Can you work these out from the model? Positions are in its coordinate system, mm. Give positions to 0.01 mm unless a question says otherwise; leave off trailing zeros. Order: outer loops, then holes, each group sorted by start corner. A loop starts at its lowest first (then second) coordinate and runs counter-clockwise, first axis right, second up. Notation, with made-up numbers: M -26.5,50.5 L -13.5,50.5 A21 cw -13.5,80.5 Z; hole C 20,-12.5 d9. An arc over 180 degrees is marked long. Write each question's results on one line, items separated by ' | '.
from build123d import *

# Parameters (mm, degrees)
SKETCH1_W           = 152.4
SKETCH1_H           = 63.5
BOSS_EXTRUDE1_DEPTH = 6.35
CUT_EXTRUDE1_REACH  = 14.7
SKETCH2_R           = 9.525


with BuildPart() as part:
    # Sketch1 → Boss-Extrude1 (new body, symmetric)
    with BuildSketch(Plane(origin=(0, 0, 0), x_dir=(0, 0, -1), z_dir=(1, 0, 0))):
        Rectangle(SKETCH1_W, SKETCH1_H)
    extrude(amount=BOSS_EXTRUDE1_DEPTH, both=True)

    # Sketch2 → Cut-Extrude1 (cut, up to next)
    with BuildSketch(Plane(origin=(6.35, 0, 0), x_dir=(0, 0, -1), z_dir=(1, 0, 0)), mode=Mode.PRIVATE) as cut_extrude1_sk1:
        with Locations((-50.8, 6.35)):
            Circle(SKETCH2_R)
    cut_extrude1_tool1 = extrude(cut_extrude1_sk1.sketch, amount=-CUT_EXTRUDE1_REACH, mode=Mode.PRIVATE) & part.part
    add(cut_extrude1_tool1.solids().sort_by_distance((6.35, 6.35, 50.8))[0], mode=Mode.SUBTRACT)


solid = part.part
(1) Imagine slicing it at C-C, the plane x = 0.75. Write out the boundary of the cut face in (y, z) (3 decimals), plus the area to 3 significant figures.
Data:
outline: M -31.75,-76.2 L 31.75,-76.2 L 31.75,76.2 L -31.75,76.2 Z; hole C 6.35,50.8 d19.05 | area: 9,390 mm2
(2) Imagine slicing it at B-B, the plane y = 6.35. Write out the boundary of the cut face in (x, z) (3 decimals), plus the area to 3 significant figures.
Data:
outline: M -6.35,-76.2 L 6.35,-76.2 L 6.35,41.275 L -6.35,41.275 Z; M -6.35,60.325 L 6.35,60.325 L 6.35,76.2 L -6.35,76.2 Z | area: 1,690 mm2
(3) Imagine slicing it at A-A, the plane z = 50.8. Write out the boundary of the cut face in (x, y) (3 decimals), plus the area to 3 significant figures.
Data:
outline: M -6.35,-31.75 L 6.35,-31.75 L 6.35,-3.175 L -6.35,-3.175 Z; M -6.35,15.875 L 6.35,15.875 L 6.35,31.75 L -6.35,31.75 Z | area: 565 mm2
(4) I need wall thicknesses on L1, parallel to Y at x = -1.75, z = 50.8 (3 decimals); L2, parallel to Z at x = -5.75, y = 12; L3, parallel to Z at x = 1.25, y = 10. Which ranges of each line are inside material? Lowest first, please. Write a range as from..to.
Data:
L1: y = -31.75..-3.175, 15.875..31.75 | L2: z = -76.2..43.13, 58.47..76.2 | L3: z = -76.2..42, 59.6..76.2
